```python
from build123d import *

# Parameters (mm, degrees)
SKETCH1_W           = 220
SKETCH1_H           = 200
BOSS_EXTRUDE1_DEPTH = 3
SKETCH3_W           = 220
SKETCH3_H           = 200
BOSS_EXTRUDE3_DEPTH = 80
SKETCH9_W           = 214
SKETCH9_H           = 194
CUT_EXTRUDE1_DEPTH  = 77
SKETCH13_W          = 194
SKETCH13_H          = 77
CUT_EXTRUDE4_DEPTH  = 197


with BuildPart() as part:
    # Sketch1 → Boss-Extrude1 (new body)
    with BuildSketch(Plane(origin=(0, 0, 0), x_dir=(1, 0, 0), z_dir=(0, 1, 0))):
        with Locations((2.493847253, -12.542456993)):
            Rectangle(SKETCH1_W, SKETCH1_H)
    extrude(amount=BOSS_EXTRUDE1_DEPTH)

    # Sketch3 → Boss-Extrude3 (add)
    with BuildSketch(Plane(origin=(0, 3, 0), x_dir=(1, 0, 0), z_dir=(0, 1, 0))):
        with Locations((2.493847253, -12.542456993)):
            Rectangle(SKETCH3_W, SKETCH3_H)
    extrude(amount=BOSS_EXTRUDE3_DEPTH)

    # Sketch9 → Cut-Extrude1 (cut)
    with BuildSketch(Plane(origin=(0, 83, 0), x_dir=(1, 0, 0), z_dir=(0, 1, 0))):
        with Locations((2.493847253, -12.542456993)):
            Rectangle(SKETCH9_W, SKETCH9_H)
    extrude(amount=-CUT_EXTRUDE1_DEPTH, mode=Mode.SUBTRACT)

    # Sketch13 → Cut-Extrude4 (cut)
    with BuildSketch(Plane.ZY.offset(-109.493847253)):
        with Locations((12.542456993, 44.5)):
            Rectangle(SKETCH13_W, SKETCH13_H)
    extrude(amount=-CUT_EXTRUDE4_DEPTH, mode=Mode.SUBTRACT)


solid = part.part
```
Can you work these out from the model? Positions are in its coordinate system, mm. A direction names the side the tool comes from. Round coordinates to 2 decimals unless told otherwise and drop trailing zeros. Loops run counter-clockwise (first coordinate to the right, second up) from the corner with the lowest first, then second, coordinate; pieces in that order, holes last. Notation, with made-up numbers: (79, 6) -> (95, 6) arc R18 ccw to (95, 21) -> close; hole circle Ø4 at (-17, 15). An arc over 180 degrees is marked (long way). Answer in a Markdown table with one row per item.
Item 1: Will this pin go through, and if not, where does the flat tip stop? P1, Ø1, axis at y = 28.5, z = -55.5, coming from the +X side.
Answer block:
| item | result |
|---|---|
| P1 | x = -104.51 |
Item 2: Suppose I cut it at C-C, the plane x = 84.5. List the corners of the cut face in (y, z) for me, plus the area to 3 significant figures.
Answer block:
| item | result |
|---|---|
| outline | (0, -87.46) -> (83, -87.46) -> (83, -84.46) -> (6, -84.46) -> (6, 109.54) -> (83, 109.54) -> (83, 112.54) -> (0, 112.54) -> close |
| area | 1,660 mm² |
Item 3: Suppose I cut it at A-A, the plane z = 100. List the corners of the cut face in (x, y) for me, plus the area to 3 significant figures.
Answer block:
| item | result |
|---|---|
| outline | (-107.51, 0) -> (112.49, 0) -> (112.49, 6) -> (-104.51, 6) -> (-104.51, 83) -> (-107.51, 83) -> close |
| area | 1,550 mm² |
Item 4: If I drill on probe 1 along Z at (x, y) = (17, 50.5); probe 2 along X at (y, z) = (58, -30.5); probe 3 along Y at (x, z) = (44, -46.5), over which ranges is the centre line in solid material (lowest first)?
Answer block:
| item | result |
|---|---|
| probe 1 | -87.46 to -84.46, 109.54 to 112.54 |
| probe 2 | -107.51 to -104.51 |
| probe 3 | 0 to 6 |
Item 5: Suppose I cut it at B-B, the plane y = 67.5. List the corners of the cut face in (x, z) for me.
Answer block:
| item | result |
|---|---|
| outline | (-107.51, -87.46) -> (112.49, -87.46) -> (112.49, -84.46) -> (-104.51, -84.46) -> (-104.51, 109.54) -> (112.49, 109.54) -> (112.49, 112.54) -> (-107.51, 112.54) -> close |
Item 6: We'd pull the mould along Z, two halves only. Please class faces 1 (the flat face through (2, 44, -84.458)), 2 (the flat face through (2, 45, 109.542)), 3 (the flat face through (1, 41, -87.458)), 4 (the flat face through (1, 0, 11)): released by +Z, released by -Z, zero draft, split by the parting line, or undercut.
Answer block:
| item | result |
|---|---|
| face 1 | undercut |
| face 2 | undercut |
| face 3 | released by -Z |
| face 4 | zero draft |
Item 7: On a 3-axis mill with a long thin cutter (end or side, diameter ignored), from which of +Z, -Z, +X, -X, +Y, -Y can I reach the whole of each face in a straight line? I mean faces 5 (the flat face through (112.494, 1, 13)), 6 (the flat face through (-104.506, 45, 14)). Say none if no direction works.
Answer block:
| item | result |
|---|---|
| face 5 | +Z, -Z, +X, +Y, -Y |
| face 6 | +X, +Y |
